Source: CAD feature listing. Evaluate the final solid. Frame: model axes, mm. Face numbers are marked on the shaded views. Round coordinates to 2 decimals unless told otherwise and drop trailing zeros. Order: outer loops, then holes, each group sorted by start corner. A loop starts at its lowest first (then second) coordinate and runs counter-clockwise, first axis right, second up. Notation, with made-up numbers: (13.25, -13.75) -> (28.25, -13.75) arc R21 ccw to (28.25, 17.25) -> close; hole circle Ø9 at (76, 11). An arc over 180 degrees is marked (long way). One line per item, written item: value. Start each with the question number.
1) Pin query (flat end, axial travel): P1, Ø2, axis at x = -1, z = -12, coming from the +Y side; P2, Ø2, axis at y = 1.5, z = -5, coming from the -X side; P3, Ø5, axis at x = 0, y = 0, coming from the -Z side (3 decimals); P4, Ø5, axis at y = -4, z = -10.5, coming from the +X side. Return the tip coordinate at first contact, or that it passes through.
2) Section B-B (z = -8.5). Return the cut outline in (x, y) (3 decimals).
3) Ray query, L1, parallel to Y at x = 0, z = -12.5 (3 decimals); L2, parallel to Z at x = -10.5, y = 9; L3, parallel to X at y = 2, z = -7.5. Return the intervals inside material, ascending.
4) Section A-A (z = -5.5). Return the cut outline in (x, y) (3 decimals).
5) Mould query, pull axis Y, two halves, no side actions, for the marked faces 1, 2 and 3. Classes: pulls with the +Y half, pulls with the -Y half, needs draft (parallel to the pull), parting line crosses it, or undercut.
```python
from build123d import *

# Parameters (mm, degrees)
F2_R     = 3.175
F3_DEPTH = 25.4
F4_R     = 3.175
F5_DEPTH = 25.4


with BuildPart() as f1:
    # F0 (on Front) → F1 (revolve)
    with BuildSketch(Plane.XZ):
        with BuildLine():
            Line((0, -19.05), (0, 0))
            Line((0, 0), (-15.24, 0))
            Line((-15.24, 0), (-15.24, -7.9375))
            ThreePointArc((-15.24, -7.9375), (-14.117468, -8.402468), (-13.6525, -9.525))
            ThreePointArc((-13.6525, -9.525), (-14.117468, -10.647532), (-15.24, -11.1125))
            Line((-15.24, -11.1125), (-15.24, -19.05))
            Line((-15.24, -19.05), (0, -19.05))
        make_face()
    revolve(axis=Axis((0, 0, -9.525), (0, 0, -1)))

    # F2 (on face) → F3 (cut)
    with BuildSketch(Plane.XY):
        Circle(F2_R)
    extrude(amount=-F3_DEPTH, mode=Mode.SUBTRACT)

    # F4 (on face) → F5 (cut)
    with BuildSketch(Plane.XY):
        Circle(F4_R)
    extrude(amount=-F5_DEPTH, mode=Mode.SUBTRACT)


solid = f1.part
```
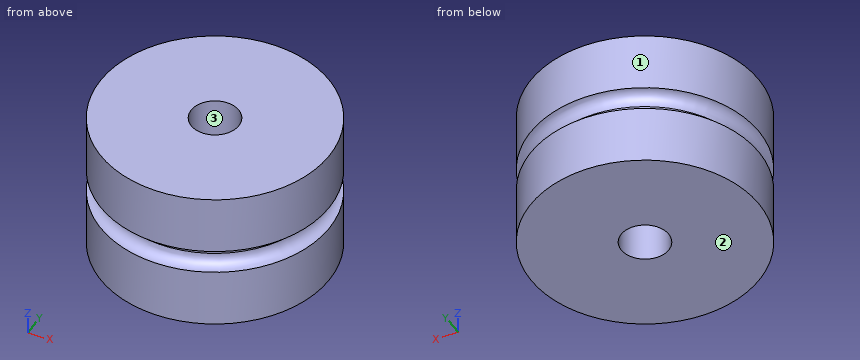
Findings:
1. P1: y = 15.24
1. P2: x = -15.23
1. P3: through
1. P4: x = 15.16
2. outline: circle Ø28.056 at (0, 0); hole circle Ø6.35 at (0, 0)
3. L1: -15.24 to -3.175, 3.175 to 15.24
3. L2: -19.05 to -10.25, -8.8 to 0
3. L3: -15.11 to -2.47, 2.47 to 15.11
4. outline: circle Ø30.48 at (0, 0); hole circle Ø6.35 at (0, 0)
5. face 1: parting line crosses it
5. face 2: needs draft
5. face 3: undercut
